Geometry: final body of the model. Coordinates: model frame, mm. A direction names the side the tool comes from. Round coordinates to 2 decimals unless told otherwise and drop trailing zeros. Write each loop counter-clockwise with the first axis right and the second up, starting at its lowest first coordinate (ties: lowest second). Pieces come first, ordered by that corner, then holes.
from build123d import *

# Parameters (mm, degrees)
SKETCH062_W         = 94.8
SKETCH062_H         = 127
PAD_DEPTH           = 28.5
POCKET011_DEPTH     = 100
SKETCH064_W         = 86.8
SKETCH064_H         = 23.38
POCKET012_DEPTH     = 25
SKETCH065_W         = 96.8
SKETCH065_H         = 129
POCKET013_DEPTH     = 3.2
SKETCH066_W         = 127
SKETCH066_H         = 3
PAD001_DEPTH        = 9
SKETCH067_W         = 127
SKETCH067_H         = 3
PAD002_DEPTH        = 9
SKETCH069_R         = 1.65
POCKET014_DEPTH     = 5
SKETCH072_W         = 90.8
SKETCH072_H         = 0.2
POCKET015_DEPTH     = 100
HOLE016_D           = 3.3
HOLE016_DEPTH       = 5
HOLE016_CSINK_D     = 6
HOLE016_CSINK_ANGLE = 90
HOLE017_D           = 3.5
HOLE017_DEPTH       = 5.3
HOLE017_CSINK_D     = 6
HOLE017_CSINK_ANGLE = 90
FILLET_R            = 3.35
FILLET002_R         = 3.35
SKETCH076_W         = 18
SKETCH076_H         = 4
POCKET017_DEPTH     = 2


with BuildPart() as part:
    # Sketch062 → Pad (new body)
    with BuildSketch(Plane.XY):
        with Locations((42.1, 73.5)):
            Rectangle(SKETCH062_W, SKETCH062_H)
    extrude(amount=PAD_DEPTH)

    # Sketch063 (on Face1 of Pad) → Pocket011 (cut)
    with BuildSketch(Plane.XZ.offset(-10)):
        Polygon((-3.299998, 2.01), (-3.299998, 6.61), (-0.299998, 6.61), (-0.299998, 25.39), (84.500002, 25.39), (84.500002, 6.61), (87.500002, 6.61), (87.500002, 2.01), align=None)
    extrude(amount=-POCKET011_DEPTH, mode=Mode.SUBTRACT)

    # Sketch064 (on Face14 of Pocket011) → Pocket012 (cut)
    with BuildSketch(Plane(origin=(0, 137, 0), x_dir=(-1, 0, 0), z_dir=(0, 1, 0))):
        with Locations((-42.1, 13.689999)):
            Rectangle(SKETCH064_W, SKETCH064_H)
    extrude(amount=-POCKET012_DEPTH, mode=Mode.SUBTRACT)

    # Sketch065 (on Face4 of Pocket012) → Pocket013 (cut)
    with BuildSketch(Plane.XY.offset(28.5)):
        with Locations((42.180762, 73.419241)):
            Rectangle(SKETCH065_W, SKETCH065_H)
    extrude(amount=-POCKET013_DEPTH, mode=Mode.SUBTRACT)

    # Sketch066 (on Face12 of Pocket013) → Pad001 (join)
    with BuildSketch(Plane(origin=(-5.3, 0, 0), x_dir=(0, -1, 0), z_dir=(-1, 0, 0))):
        with Locations((-73.5, 23.8)):
            Rectangle(SKETCH066_W, SKETCH066_H)
    extrude(amount=PAD001_DEPTH)

    # Sketch067 (on Face3 of Pad001) → Pad002 (join)
    with BuildSketch(Plane.YZ.offset(89.5)):
        with Locations((73.500002, 23.8)):
            Rectangle(SKETCH067_W, SKETCH067_H)
    extrude(amount=PAD002_DEPTH)

    # Sketch069 (on Face17 of Pad002) → Pocket014 (cut)
    with BuildSketch(Plane.XY.offset(25.3)):
        with Locations((-9.8, 20.000492)):
            Circle(SKETCH069_R)
        with Locations((-9.8, 46.749416)):
            Circle(SKETCH069_R)
        with Locations((-9.8, 73.500001)):
            Circle(SKETCH069_R)
        with Locations((-9.8, 100.249657)):
            Circle(SKETCH069_R)
        with Locations((-9.8, 126.999153)):
            Circle(SKETCH069_R)
        with Locations((94, 20.001339)):
            Circle(SKETCH069_R)
        with Locations((94, 46.750263)):
            Circle(SKETCH069_R)
        with Locations((94, 73.500848)):
            Circle(SKETCH069_R)
        with Locations((94, 100.250504)):
            Circle(SKETCH069_R)
        with Locations((94, 127)):
            Circle(SKETCH069_R)
    extrude(amount=-POCKET014_DEPTH, mode=Mode.SUBTRACT)

    # Sketch072 (on Face1 of Pocket014) → Pocket015 (cut)
    with BuildSketch(Plane.XZ.offset(-10)):
        with Locations((42.099998, 1.91)):
            Rectangle(SKETCH072_W, SKETCH072_H)
    extrude(amount=-POCKET015_DEPTH, mode=Mode.SUBTRACT)

    # Hole016
    with Locations(Plane(origin=(84.500002, 0, 0), x_dir=(0, -1, 0), z_dir=(-1, 0, 0))):
        with Locations((-33.375, 18.05)):
            CounterSinkHole(HOLE016_D / 2, HOLE016_CSINK_D / 2, depth=HOLE016_DEPTH, counter_sink_angle=HOLE016_CSINK_ANGLE)

    # Hole017
    with Locations(Plane.YZ):
        with Locations((33.374271, 18.355644)):
            CounterSinkHole(HOLE017_D / 2, HOLE017_CSINK_D / 2, depth=HOLE017_DEPTH, counter_sink_angle=HOLE017_CSINK_ANGLE)

    # Fillet
    fillet_edges = [part.edges().sort_by_distance(p)[0] for p in [
        (98.5, 137.000002, 23.8),
        (-14.3, 137, 23.8),
    ]]
    fillet(fillet_edges, radius=FILLET_R)

    # Fillet002
    fillet002_edges = [part.edges().sort_by_distance(p)[0] for p in [
        (89.5, 137, 11.15),
        (-5.3, 137, 11.15),
    ]]
    fillet(fillet002_edges, radius=FILLET002_R)

    # Sketch076 (on Face40 of Fillet002) → Pocket017 (cut)
    with BuildSketch(Plane(origin=(0, 112, 0), x_dir=(-1, 0, 0), z_dir=(0, 1, 0))):
        with Locations((-15.819999, 14.3)):
            Rectangle(SKETCH076_W, SKETCH076_H)
    extrude(amount=-POCKET017_DEPTH, mode=Mode.SUBTRACT)


with BuildPart() as part_1:
    # Body008 placement: moved
    add(part.part.moved(Location((-143, 0, 0))))


solid = part_1.part
1) First-contact query: P1, Ø3, axis at x = -133, z = 3, coming from the -Y side; P2, Ø3, axis at y = 33.37, z = 18.36, coming from the -X side; P3, Ø2, axis at x = -49, y = 20, coming from the -Z side; P4, Ø6, axis at y = 39, z = 13, coming from the -X side. Flat tips, straight axial feed; report the tip coordinate or a pass-through.
2) Line query: probe 1 along Y at (x, z) = (-49, 24.2); probe 2 along X at (y, z) = (127, 23.5). Output: solid intervals per line, ascending.
3) Section C-C on y = 117.5. Output: boundary loops of the cut face in (x, z).
4) Reachability of faces 1 (the flat face through (-145, 59, 6.61)), 2 (the flat face through (-144.3, 125, 13)), 3 (the cylindrical face through (-55.299, 32.159, 19.165)) from +Z, -Z, +X, -X, +Y, -Y: full face, straight path, thin tool, end or side. Return the list, or none.
5) Section A-A on x = -116.5. Output: boundary loops of the cut face in (y, z), plus the area to 3 significant figures.
6) Draft query along X for faces 4 (the flat face through (-55.5, 59, 4)), 5 (the flat face through (-49, 10, 24)), 6 (the cylindrical face through (-50.216, 74.616, 23.821)), 7 (the flat face through (-157.3, 73, 24)). Return one class per face: pulls with the +X half, pulls with the -X half, needs draft (parallel to the pull), parting line crosses it, or undercut.
Filled in:
1. P1: stops at y = 10
1. P2: stops at x = -57.31
1. P3: passes through
1. P4: stops at x = -148.3
2. probe 1: y = 10 to 18.35, 21.65 to 45.1, 48.4 to 71.85, 75.15 to 98.6, 101.9 to 125.35, 128.65 to 137
2. probe 2: x = -157.3 to -154.45, -151.15 to -144.3, -57.5 to -50.65, -47.35 to -44.5
3. outline: (-157.3, 22.3) - (-148.3, 22.3) - (-148.3, 0) - (-53.5, 0) - (-53.5, 22.3) - (-44.5, 22.3) - (-44.5, 25.3) - (-57.5, 25.3) - (-57.5, 2) - (-144.3, 2) - (-144.3, 25.3) - (-157.3, 25.3) - close
4. face 1: -Y
4. face 2: +Z, +Y
4. face 3: +X
5. outline: (10, 0) - (137, 0) - (137, 2) - (112, 2) - (112, 25.3) - (110, 25.3) - (110, 1.81) - (10, 1.81) - close
5. area: 282 mm2
6. face 4: undercut
6. face 5: needs draft
6. face 6: undercut
6. face 7: pulls with the -X half
